Autodesk Inventor part; units mm, degrees
ref_plane "YZ Plane" through (0, 0, 0) normal (1, 0, 0) x (0, 1, 0)
ref_plane "XZ Plane" through (0, 0, 0) normal (0, 1, 0) x (-1, 0, 0)
ref_plane "XY Plane" through (0, 0, 0) normal (0, 0, 1) x (1, 0, 0)
sketch "Sketch1" plane through (0, 0, 0) normal (0, 1, 0) x (-1, 0, 0)
  circle A0 centre (0, 0) radius 28.3845
  circle A1 centre (0, 0) radius 6.35
  dimension "d0" = 56.769
  dimension "d1" = 12.7
extrude "Extrusion1" add sketch "Sketch1" along normal blind 12.7
sketch "Sketch2" plane through (0, 12.7, 0) normal (0, 1, 0) x (1, 0, 0)
  circle A0 centre (0, 0) radius 26.9875
  circle A1 centre (0, 0) radius 6.35
  dimension "d4" = 53.975
extrude "Extrusion2" add sketch "Sketch2" along normal blind 4.191
sketch "Sketch3" plane through (0, 16.891, 0) normal (0, 1, 0) x (1, 0, 0)
  line L0 (9.4957, 15.6943) -> (18.3395, -0.3764)
  line L1 (18.3395, -0.3764) -> (8.8438, -16.0707)
  line L2 (8.8438, -16.0707) -> (-9.4957, -15.6943)
  line L3 (-9.4957, -15.6943) -> (-18.3395, 0.3764)
  line L4 (-18.3395, 0.3764) -> (-8.8438, 16.0707)
  line L5 (-8.8438, 16.0707) -> (9.4957, 15.6943)
  circle A0 centre (0, 0) radius 6.35
extrude "Extrusion3" add sketch "Sketch3" along normal blind 8.89
sketch "Sketch4" plane through (0, 25.781, 0) normal (0, 1, 0) x (1, 0, 0)
  line L0 (-12.192, -12.192) -> (12.192, -12.192)
  line L1 (12.192, -12.192) -> (12.192, 12.192)
  line L2 (12.192, 12.192) -> (-12.192, 12.192)
  line L3 (-12.192, 12.192) -> (-12.192, -12.192)
  circle A0 centre (0, 0) radius 6.35
  dimension "d9" = 24.384
  dimension "d10" = 24.384
extrude "Extrusion4" add sketch "Sketch4" along normal blind 14.224
fillet "Fillet1" radius 6.35 4 edges at (12.192, 32.893, 12.192) (12.192, 32.893, -12.192) (-12.192, 32.893, -12.192) (-12.192, 32.893, 12.192)
properties part number "Top"
Model file for the job. Use its own axes, mm. A direction names the side the tool comes from. Coordinates: 2 decimals unless noted, no trailing zeros. Order: outer loops, then holes, each group sorted by start corner. A loop starts at its lowest first (then second) coordinate and runs counter-clockwise, first axis right, second up. Notation, with made-up numbers: (-28, 86) - (5, 86) arc R26 ccw to (5, 109) - close; hole circle Ø7 at (1, 41). An arc over 180 degrees is marked (long way). Return JSON: item names as keys, results as strings. Group by question number.
1) Saw through at B-B, the plane x = 24. Write the cut outline in (y, z), plus the area to 3 significant figures.
2) Tool access for faces 1 (the cylindrical face through (10.381, 32.793, 10.282)), 2 (the cylindrical face through (-10.282, 32.793, 10.381)), 3 (the cylindrical face through (10.282, 32.793, -10.381)), 4 (the cylindrical face through (-10.381, 32.793, -10.282)): list every direction of +Z, -Z, +X, -X, +Y, -Y with a clear straight run to the whole face (end or side of a thin tool).
3) Saw through at C-C, the plane z = 21. Write the cut outline in (x, y).
4) Saw through at A-A, the plane y = 34.5. Write the cut outline in (x, z), plus the area to 3 significant figures.
5) Flat gauge pins, fed straight in: P1, Ø10, axis at y = 16.5, z = 14, coming from the -X side; P2, Ø13, axis at y = 36.5, z = -2.5, coming from the +X side; P3, Ø1, axis at x = 13, z = 18.5, coming from the +Y side; P4, Ø10, axis at x = 0, z = 0, coming from the -Y side. Where does each tip first touch, or does it go through?
6) Saw through at D-D, the plane y = 4. Write the cut outline in (x, z).
7) Probe line 1 (Z direction, x = 0, y = 36.75); line 2 (X direction, y = 8, z = -5). List the from-to ranges inside material, lowest first. Write a range as from..to.
Values found:
{
 "1": {"outline": "(0, -15.16) - (12.7, -15.16) - (12.7, -12.34) - (16.89, -12.34) - (16.89, 12.34) - (12.7, 12.34) - (12.7, 15.16) - (0, 15.16) - close", "area": "488 mm²"},
 "2": {"face 1": "+Z, +X, +Y", "face 2": "+Z, -X, +Y", "face 3": "-Z, +X, +Y", "face 4": "-Z, -X, +Y"},
 "3": {"outline": "(-19.1, 0) - (19.1, 0) - (19.1, 12.7) - (16.95, 12.7) - (16.95, 16.89) - (-16.95, 16.89) - (-16.95, 12.7) - (-19.1, 12.7) - close"},
 "4": {"outline": "(-12.19, -5.84) arc R6.35 ccw to (-5.84, -12.19) - (5.84, -12.19) arc R6.35 ccw to (12.19, -5.84) - (12.19, 5.84) arc R6.35 ccw to (5.84, 12.19) - (-5.84, 12.19) arc R6.35 ccw to (-12.19, 5.84) - close; hole circle Ø12.7 at (0, 0)", "area": "433 mm²"},
 "5": {"P1": "stops at x = -26.27", "P2": "stops at x = 12.19", "P3": "stops at y = 16.89", "P4": "passes through"},
 "6": {"outline": "circle Ø56.77 at (0, 0); hole circle Ø12.7 at (0, 0)"},
 "7": {"line 1": "z = -12.19..-6.35, 6.35..12.19", "line 2": "x = -27.94..-3.91, 3.91..27.94"}
}
